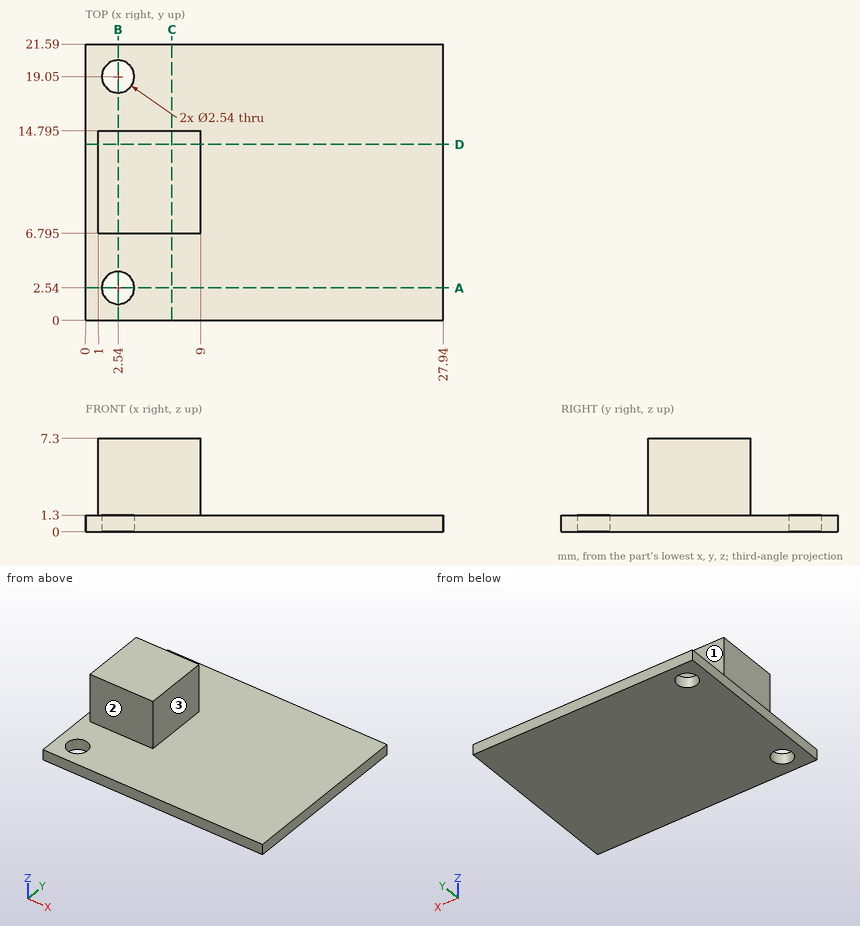
Geometry check sheet. Reference: drawing and pictorial views, mm from the part's lowest x, y, z. A direction names the side the tool comes from. Give positions to 0.01 mm unless a question says otherwise; leave off trailing zeros. Write each loop counter-clockwise with the first axis right and the second up, starting at its lowest first coordinate (ties: lowest second). Pieces come first, ordered by that corner, then holes. Notation, with made-up numbers: (-26.5, 6.5) - (21.5, 6.5) arc R16 cw to (21.5, 33.5) - close; hole circle Ø9 at (47.25, 70). An arc over 180 degrees is marked (long way). Use a Markdown table: item, result.
Q1. Section check C-C, the plane x = 6.75. Enter the section's corners in (y, z) (3 decimals).
Computed:
| item | result |
|---|---|
| outline | (0, 0) - (21.59, 0) - (21.59, 1.3) - (14.795, 1.3) - (14.795, 7.3) - (6.795, 7.3) - (6.795, 1.3) - (0, 1.3) - close |
Q2. Set-up check for the marked faces 1, 2 and 3: record each of +Z, -Z, +X, -X, +Y, -Y from which the full face is reachable in a straight line by a thin tool's end or side.
Computed:
| item | result |
|---|---|
| face 1 | +Z, +X, -X, +Y |
| face 2 | +Z, +X, -X, -Y |
| face 3 | +Z, +X, +Y, -Y |
Q3. Section check B-B, the plane x = 2.54. Enter the section's corners in (y, z) (3 decimals).
Computed:
| item | result |
|---|---|
| outline | (0, 0) - (1.27, 0) - (1.27, 1.3) - (0, 1.3) - close; (3.81, 0) - (17.78, 0) - (17.78, 1.3) - (14.795, 1.3) - (14.795, 7.3) - (6.795, 7.3) - (6.795, 1.3) - (3.81, 1.3) - close; (20.32, 0) - (21.59, 0) - (21.59, 1.3) - (20.32, 1.3) - close |
Q4. Section check A-A, the plane y = 2.54. Enter the section's corners in (x, z).
Computed:
| item | result |
|---|---|
| outline | (0, 0) - (1.27, 0) - (1.27, 1.3) - (0, 1.3) - close; (3.81, 0) - (27.94, 0) - (27.94, 1.3) - (3.81, 1.3) - close |
Q5. Section check D-D, the plane y = 13.75. Enter the section's corners in (x, z).
Computed:
| item | result |
|---|---|
| outline | (0, 0) - (27.94, 0) - (27.94, 1.3) - (9, 1.3) - (9, 7.3) - (1, 7.3) - (1, 1.3) - (0, 1.3) - close |
Q6. Thickness scan on L1, parallel to Y at x = 2.54, z = 0.4; L2, parallel to Z at x = 26.5, y = 9.25; L3, parallel to X at y = 7.75, z = 6.5. Record the ranges inside material, lowest first. Write a range as [from, to].
Computed:
| item | result |
|---|---|
| L1 | y = [0, 1.27], [3.81, 17.78], [20.32, 21.59] |
| L2 | z = [0, 1.3] |
| L3 | x = [1, 9] |
Q7. Go/stop test with flat-tipped pins: P1, Ø10, axis at x = 20, y = 5.5, coming from the +Z side; P2, Ø3, axis at x = 5, z = 4.5, coming from the +Y side (3 decimals). Record where each tip stops, or that it passes through.
Computed:
| item | result |
|---|---|
| P1 | stops at z = 1.3 |
| P2 | stops at y = 14.795 |
